from build123d import *

# Parameters (mm, degrees)
F0_W     = 406.4
F0_H     = 47.625
F1_DEPTH = 12.7
F3_DEPTH = 25.4


with BuildPart() as f1:
    # F0 (on Front) → F1 (new body)
    with BuildSketch(Plane.XZ):
        with Locations((203.2, 23.8125)):
            Rectangle(F0_W, F0_H)
    extrude(amount=F1_DEPTH)

    # F2 (on face) → F3 (cut)
    with BuildSketch(Plane.XZ.offset(12.7)):
        with BuildLine():
            Line((12.7, 47.625), (0, 47.625))
            Line((0, 47.625), (0, 34.925))
            Line((0, 34.925), (7.768212, 34.925))
            ThreePointArc((7.768212, 34.925), (8.898713, 34.581488), (9.646988, 33.667095))
            ThreePointArc((9.646988, 33.667095), (15.034867, 32.590133), (13.957905, 37.978012))
            ThreePointArc((13.957905, 37.978012), (13.043512, 38.726287), (12.7, 39.856788))
            Line((12.7, 39.856788), (12.7, 47.625))
        make_face()
        with BuildLine():
            Line((0, 12.7), (0, 0))
            Line((0, 0), (12.7, 0))
            Line((12.7, 0), (12.7, 7.768212))
            ThreePointArc((12.7, 7.768212), (13.043512, 8.898713), (13.957905, 9.646988))
            ThreePointArc((13.957905, 9.646988), (15.034867, 15.034867), (9.646988, 13.957905))
            ThreePointArc((9.646988, 13.957905), (8.898713, 13.043512), (7.768212, 12.7))
            Line((7.768212, 12.7), (0, 12.7))
        make_face()
        with BuildLine():
            Line((406.4, 12.7), (398.631788, 12.7))
            ThreePointArc((398.631788, 12.7), (397.501287, 13.043512), (396.753012, 13.957905))
            ThreePointArc((396.753012, 13.957905), (391.365133, 15.034867), (392.442095, 9.646988))
            ThreePointArc((392.442095, 9.646988), (393.356488, 8.898713), (393.7, 7.768212))
            Line((393.7, 7.768212), (393.7, 0))
            Line((393.7, 0), (406.4, 0))
            Line((406.4, 0), (406.4, 12.7))
        make_face()
        with BuildLine():
            ThreePointArc((392.442095, 37.978012), (391.365133, 32.590133), (396.753012, 33.667095))
            ThreePointArc((396.753012, 33.667095), (397.501287, 34.581488), (398.631788, 34.925))
            Line((398.631788, 34.925), (406.4, 34.925))
            Line((406.4, 34.925), (406.4, 47.625))
            Line((406.4, 47.625), (393.7, 47.625))
            Line((393.7, 47.625), (393.7, 39.856788))
            ThreePointArc((393.7, 39.856788), (393.356488, 38.726287), (392.442095, 37.978012))
        make_face()
    extrude(amount=-F3_DEPTH, mode=Mode.SUBTRACT)


solid = f1.part
For this review, take the finished solid that the model builds, in its own axes (mm). A direction names the side the tool comes from. Round coordinates to 2 decimals unless told otherwise and drop trailing zeros. Write each loop counter-clockwise with the first axis right and the second up, starting at its lowest first coordinate (ties: lowest second). Pieces come first, ordered by that corner, then holes. Notation, with made-up numbers: (-19.75, 4.25) - (4.25, 4.25) arc R23 ccw to (4.25, 22.25) - close; hole circle Ø10 at (82, 71). An arc over 180 degrees is marked (long way). Use a Markdown table: item, result.
Q1. Clearance check with flat-ended pins moving along their axes: pin 1 (4 mm diameter, centred on x = 12.7, z = 12.7, fed in from -Y); pin 2 (4 mm diameter, centred on y = -5, z = 5.5, fed in from -X); pin 3 (6 mm diameter, centred on y = -8.5, z = 42.5, fed in from +X); pin 4 (4 mm diameter, centred on x = 402.5, y = -6.5, fed in from +Z) (3 decimals). State where each tip first meets the part, or that it passes through.
Derived:
| item | result |
|---|---|
| pin 1 | passes through |
| pin 2 | stops at x = 12.7 |
| pin 3 | stops at x = 393.7 |
| pin 4 | stops at z = 34.925 |
Q2. The part is to be moulded in two halves that separate along X. For faces 1 (the flat face through (200, 0, 24)), 2 (the flat face through (406.4, -6, 24)), 3 (the cylindrical face through (14.97, -6.439, 32.527)), say which applies: pulls with the +X half, pulls with the -X half, needs draft (parallel to the pull), parting line crosses it, or undercut.
Derived:
| item | result |
|---|---|
| face 1 | needs draft |
| face 2 | pulls with the +X half |
| face 3 | undercut |
Q3. We need section A-A (y = -9.25). Give the boundary of the cut face in (x, z) (3 decimals).
Derived:
| item | result |
|---|---|
| outline | (0, 12.7) - (7.768, 12.7) arc R2.032 ccw to (9.647, 13.958) arc R3.302 cw (long way) to (13.958, 9.647) arc R2.032 ccw to (12.7, 7.768) - (12.7, 0) - (393.7, 0) - (393.7, 7.768) arc R2.032 ccw to (392.442, 9.647) arc R3.302 cw (long way) to (396.753, 13.958) arc R2.032 ccw to (398.632, 12.7) - (406.4, 12.7) - (406.4, 34.925) - (398.632, 34.925) arc R2.032 ccw to (396.753, 33.667) arc R3.302 cw (long way) to (392.442, 37.978) arc R2.032 ccw to (393.7, 39.857) - (393.7, 47.625) - (12.7, 47.625) - (12.7, 39.857) arc R2.032 ccw to (13.958, 37.978) arc R3.302 cw (long way) to (9.647, 33.667) arc R2.032 ccw to (7.768, 34.925) - (0, 34.925) - close |
Q4. Wall thickness on line 1 along X through (y, z) = (-6, 33); line 2 along X through (y, z) = (-4.25, 4.5); line 3 along X through (y, z) = (-5.75, 39): over which ranges is each line inside the solid? List them lowest first.
Derived:
| item | result |
|---|---|
| line 1 | x = 0 to 10.02, 15.38 to 391.02, 396.38 to 406.4 |
| line 2 | x = 12.7 to 393.7 |
| line 3 | x = 12.89 to 393.51 |
Q5. Machinability: for faces 4 (the flat face through (403, -6, 12.7)), 5 (the flat face through (4, -6, 34.925)), 6 (the cylindrical face through (391.43, -6.44, 15.1)), 7 (the flat face through (12.7, -6, 4)), 8 (the flat face through (402, -6, 34.925)), which of the approach directions +Z, -Z, +X, -X, +Y, -Y give a long, thin tool a straight path to every point of the face, cutting with its end or side? Answer none if there is none.
Derived:
| item | result |
|---|---|
| face 4 | -Z, +X, +Y, -Y |
| face 5 | +Z, -X, +Y, -Y |
| face 6 | +Y, -Y |
| face 7 | -Z, -X, +Y, -Y |
| face 8 | +Z, +X, +Y, -Y |
